Could you check a few things on this drawing? It's one solid part, dimensions in mm from its lowest x, y, z. A direction names the side the tool comes from. Give positions to 0.01 mm unless a question says otherwise; leave off trailing zeros. Order: outer loops, then holes, each group sorted by start corner. A loop starts at its lowest first (then second) coordinate and runs counter-clockwise, first axis right, second up.
Item 1: I want a section at B-B, the plane x = 3. Write out the boundary of the cut face in (y, z).
Item 2: I want a section at C-C, the plane y = 43. Write out the boundary of the cut face in (x, z).
Item 3: If I drill on line 1 along X through (y, z) = (25.5, 18.5); line 2 along Y through (x, z) = (3, 14); line 3 along Y through (x, z) = (18.5, 20), over which ranges is the centre line in solid material (lowest first)?
Item 4: I want a section at D-D, the plane z = 5. Write out the boundary of the cut face in (x, y) (1 decimal), then the cut area to 3 significant figures.
Item 5: I want a section at A-A, the plane z = 18.5. Write out the boundary of the cut face in (x, y), then the cut area to 3 significant figures.
Item 6: I'm going to push flat-ended pins straight in: pin 1 Ø2.5 at (x, z) = (25.5, 5.5) entering from -Y; pin 2 Ø3.5 at (x, z) = (15.5, 26.5) entering from -Y; pin 3 Ø0.9 at (x, z) = (33.5, 18) entering from -Y; pin 4 Ø3 at (y, z) = (36.5, 7) entering from -X (1 decimal). Where does each tip first touch, or does it pass through?
Item 7: Which directions (+Z, -Z, +X, -X, +Y, -Y) give clear straight access to the entire face, cutting with the end or side of a thin tool? Please do the marked faces 1, 2 and 3.
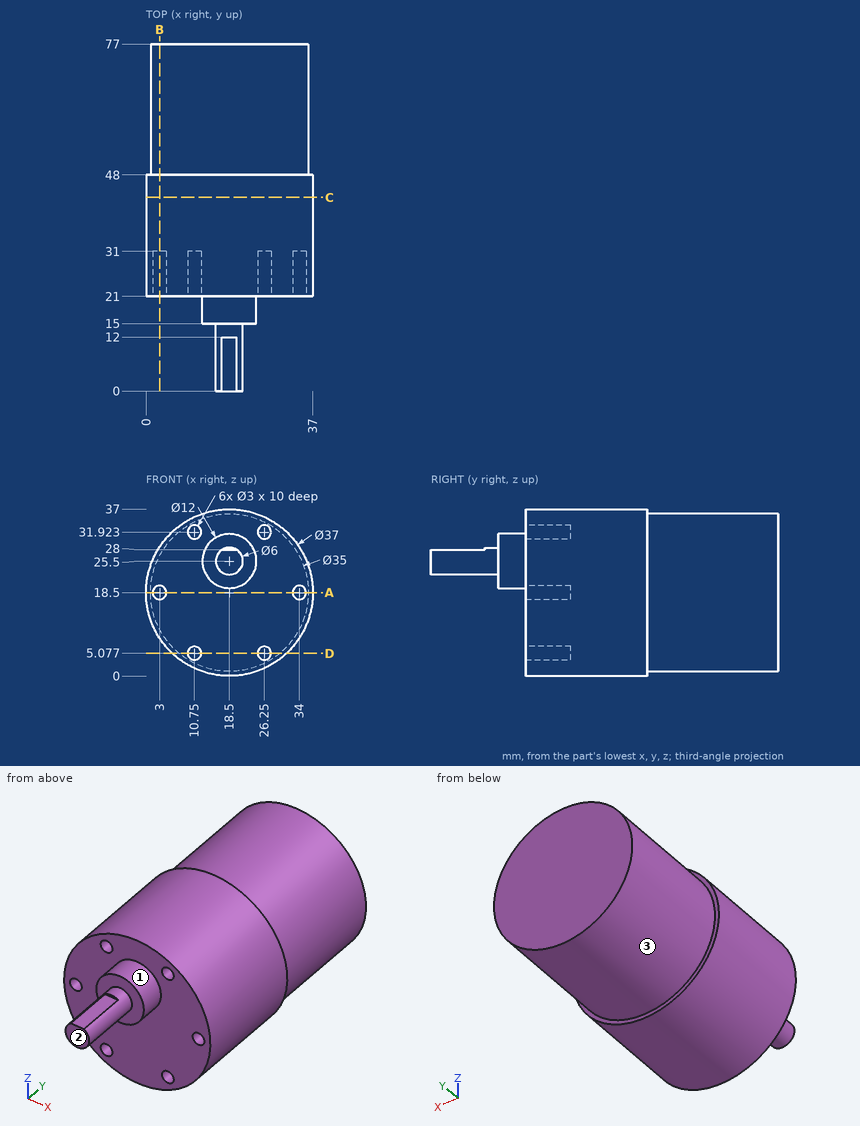
Results list:
1. outline: (21, 8.4) - (48, 8.4) - (48, 10.38) - (77, 10.38) - (77, 26.62) - (48, 26.62) - (48, 28.6) - (21, 28.6) - (21, 20) - (31, 20) - (31, 17) - (21, 17) - close
2. outline: circle Ø37 at (18.5, 18.5)
3. line 1: x = 0 to 1.5, 4.5 to 32.5, 35.5 to 37
3. line 2: y = 21 to 77
3. line 3: y = 15 to 77
4. outline: (5.9, 21) - (9.3, 21) - (9.3, 31) - (12.2, 31) - (12.2, 21) - (24.8, 21) - (24.8, 31) - (27.7, 31) - (27.7, 21) - (31.1, 21) - (31.1, 48) - (29.6, 48) - (29.6, 77) - (7.4, 77) - (7.4, 48) - (5.9, 48) - close
4. area: 1,270 mm2
5. outline: (0, 21) - (1.5, 21) - (1.5, 31) - (4.5, 31) - (4.5, 21) - (32.5, 21) - (32.5, 31) - (35.5, 31) - (35.5, 21) - (37, 21) - (37, 48) - (36, 48) - (36, 77) - (1, 77) - (1, 48) - (0, 48) - close
5. area: 1,950 mm2
6. pin 1: stops at y = 21
6. pin 2: stops at y = 0
6. pin 3: stops at y = 31
6. pin 4: stops at x = 2.9
7. face 1: -Y
7. face 2: +Z, -Z, +X, -X, -Y
7. face 3: +Y
